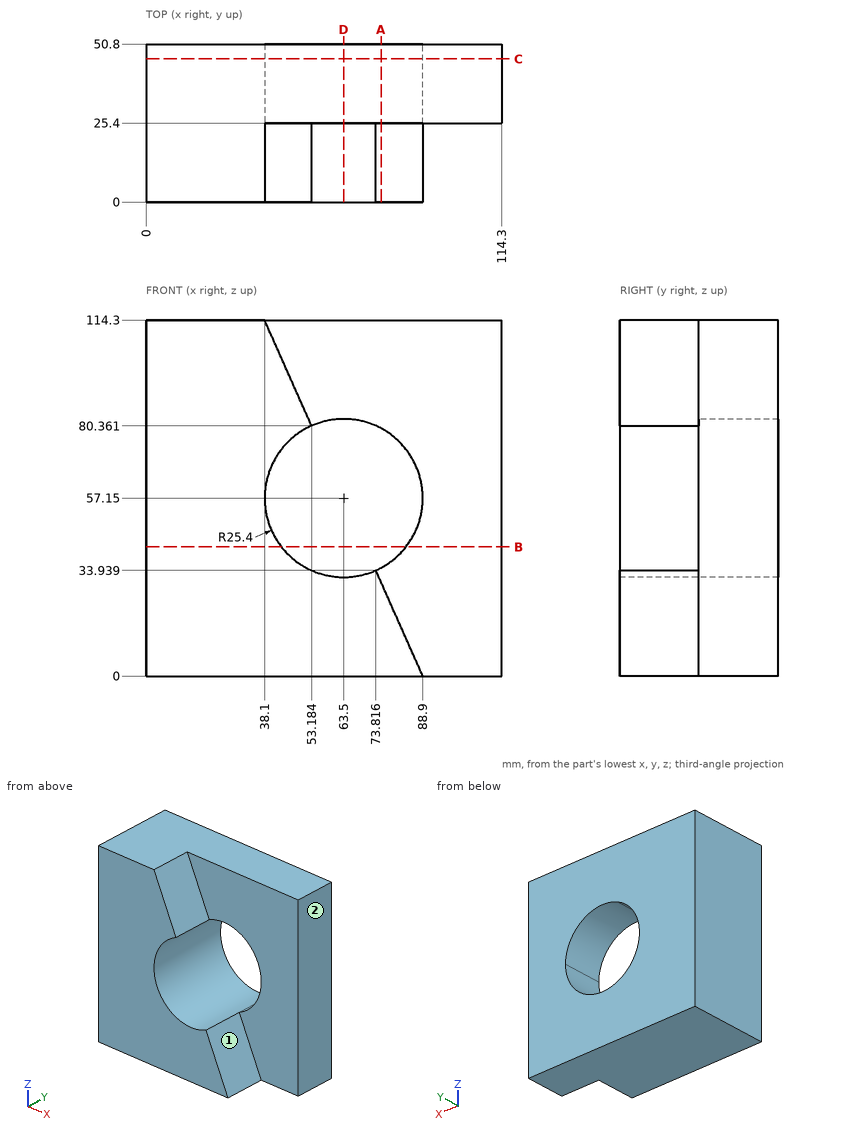
The figure shows three views and two pictorial views of one solid part (mm, origin at its lowest corner). Answer the questions. A direction names the side the tool comes from. Round coordinates to 2 decimals unless told otherwise and drop trailing zeros. Order: outer loops, then holes, each group sorted by start corner. A loop starts at its lowest first (then second) coordinate and runs counter-clockwise, first axis right, second up. Notation, with made-up numbers: (73, -34.75) -> (125, -34.75) arc R30 ccw to (125, -11.75) -> close; hole circle Ø3 at (-22, 0). An arc over 180 degrees is marked (long way). One line per item, written item: value.
Item 1: Find section A-A, the plane x = 75.5. Give the vertices of the cut face in (y, z), then the cut area to 3 significant figures.
Taken from the geometry:
outline: (0, 0) -> (50.8, 0) -> (50.8, 34.76) -> (25.4, 34.76) -> (25.4, 30.15) -> (0, 30.15) -> close; (25.4, 79.54) -> (50.8, 79.54) -> (50.8, 114.3) -> (25.4, 114.3) -> close
area: 2,530 mm2
Item 2: Given P1, Ø3, axis at y = 14, z = 85.5, coming from the +X side, flat-ended and moving along its own axis, determine where the tip first touches the part or whether it passes through.
Taken from the geometry:
P1: stops at x = 51.57
Item 3: Find section B-B, the plane z = 41.5. Give the vertices of the cut face in (x, y).
Taken from the geometry:
outline: (0, 0) -> (43.49, 0) -> (43.49, 50.8) -> (0, 50.8) -> close; (83.51, 25.4) -> (114.3, 25.4) -> (114.3, 50.8) -> (83.51, 50.8) -> close
Item 4: Straight lines are drawn through the part: L1, parallel to Y at x = 64, z = 89.5; L2, parallel to X at y = 26, z = 44.5; L3, parallel to X at y = 35.5, z = 78 (1 decimal). For each, find the intervals that lie inside material, in ascending order.
Taken from the geometry:
L1: y = 25.4 to 50.8
L2: x = 0 to 41.47, 85.53 to 114.3
L3: x = 0 to 49, 78 to 114.3
Item 5: For the marked faces 1 and 2, determine the directions among +Z, -Z, +X, -X, +Y, -Y from which every point of the face is accessible in a straight line to the end or side of a thin tool.
Taken from the geometry:
face 1: +Z, +X, -Y
face 2: +Z, -Z, +X, +Y, -Y
Item 6: Find section C-C, the plane y = 46. Give the vertices of the cut face in (x, z).
Taken from the geometry:
outline: (0, 0) -> (114.3, 0) -> (114.3, 114.3) -> (0, 114.3) -> close; hole (73.82, 33.94) arc R25.4 ccw to (88.9, 57.15) arc R25.4 ccw (long way) to start
Item 7: Find section D-D, the plane x = 63.5. Give the vertices of the cut face in (y, z), then the cut area to 3 significant figures.
Taken from the geometry:
outline: (0, 0) -> (50.8, 0) -> (50.8, 31.75) -> (0, 31.75) -> close; (25.4, 82.55) -> (50.8, 82.55) -> (50.8, 114.3) -> (25.4, 114.3) -> close
area: 2,420 mm2
